Build history of the part. All positions in model axes, mm. Round coordinates to 2 decimals unless told otherwise and drop trailing zeros. Loops run counter-clockwise (first coordinate to the right, second up) from the corner with the lowest first, then second, coordinate; pieces in that order, holes last. Notation, with made-up numbers: (72.5, 63.25) - (80.5, 63.25) arc R14 ccw to (80.5, 82.25) - close; hole circle Ø5 at (-8.5, 4). An arc over 180 degrees is marked (long way). Put each result on its own line as item: value. Start each with the question number.
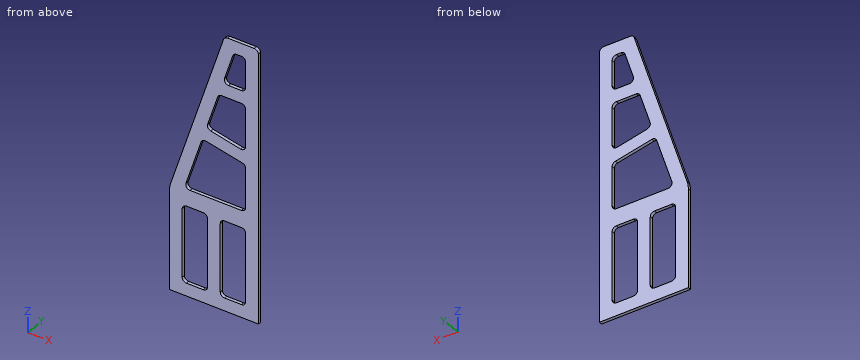
from build123d import *

# Parameters (mm, degrees)
F0_W     = 152.4
F0_H     = 457.2
F1_DEPTH = 19.05
F2_R     = 25.4
F4_R     = 152.4


# Not quite as in the source:
# - two fillets or chamfers of one size are made in one step


with BuildPart() as f1:
    # F0 (on Front) → F1 (new body)
    with BuildSketch(Plane.XZ):
        Polygon((266.7, -812.8), (266.7, 812.8), (63.5, 812.8), (-266.7, -203.2), (-266.7, -812.8), align=None)
        with Locations((-114.3, -508)):
            Rectangle(F0_W, F0_H, mode=Mode.SUBTRACT)
        with Locations((114.3, -508)):
            Rectangle(F0_W, F0_H, mode=Mode.SUBTRACT)
        Polygon((190.5, -177.8), (-178.3216873813, -177.8), (-79.2616873813, 127), (-69.7940460934, 156.1312039627), (190.5, 101.6), align=None, mode=Mode.SUBTRACT)
        Polygon((190.5, 457.2), (190.5, 228.6), (190.5, 177.8), (-46.2416873813, 228.6), (28.0533126187, 457.2), align=None, mode=Mode.SUBTRACT)
        Polygon((118.67604537, 736.6), (190.5, 736.6), (190.5, 533.4), (52.8183126187, 533.4), align=None, mode=Mode.SUBTRACT)
    extrude(amount=F1_DEPTH)

    # F2
    f2_edges = [f1.edges().sort_by_distance(p)[0] for p in [
        (28.053313, -9.525, 457.2),
        (-178.321687, -9.525, -177.8),
        (-190.5, -9.525, -279.4),
        (38.1, -9.525, -279.4),
        (-38.1, -9.525, -279.4),
        (190.5, -9.525, -279.4),
        (190.5, -9.525, 457.2),
        (190.5, -9.525, -177.8),
        (-190.5, -9.525, -736.6),
        (38.1, -9.525, -736.6),
        (-38.1, -9.525, -736.6),
        (190.5, -9.525, -736.6),
        (190.5, -9.525, 533.4),
        (266.7, -9.525, 812.8),
        (52.818313, -9.525, 533.4),
        (190.5, -9.525, 736.6),
        (118.676045, -9.525, 736.6),
        (190.5, -9.525, 177.8),
        (-46.241687, -9.525, 228.6),
        (-69.794046, -9.525, 156.131204),
        (190.5, -9.525, 101.6),
        (63.5, -9.525, 812.8),
    ]]
    fillet(f2_edges, radius=F2_R)

    # F4
    f4_edges = [f1.edges().sort_by_distance(p)[0] for p in [
        (-266.7, -9.525, -203.2),
    ]]
    fillet(f4_edges, radius=F4_R)


solid = f1.part
Item 1: Slice it at A-A (z = -631.5). Give the cut face in (x, y).
Item 2: Slice it at C-C (y = -13). Give the number of separate pieces and of enclosed holes in the cut face, plus the area to 3 significant figures.
Item 3: Slice it at D-D (z = 37.5). Give the cut face in (x, y), plus the area to 3 significant figures.
Item 4: Slice it at B-B (z = 650). Give the cut face in (x, y), plus the area to 3 significant figures.
Item 5: Drop flat-ended pins along their axis: pin 1 Ø9.5 at (y, z) = (-12.5, -84.5) entering from -X; pin 2 Ø8 at (y, z) = (-16.5, 541.5) entering from -X; pin 3 Ø9.5 at (y, z) = (-7.5, 311) entering from -X. Give the stop position or say it passes through.
Item 6: Drill centre lines: probe 1 along X at (y, z) = (-15.5, -486); probe 2 along Z at (x, y) = (150, -13); probe 3 along Z at (x, y) = (157.5, -6.5). Where is each one in solid material? Low to high. Write a range as [from, to].
Computed values:
1. outline: (-266.7, -19.05) - (-190.5, -19.05) - (-190.5, 0) - (-266.7, 0) - close; (-38.1, -19.05) - (38.1, -19.05) - (38.1, 0) - (-38.1, 0) - close; (190.5, -19.05) - (266.7, -19.05) - (266.7, 0) - (190.5, 0) - close
2. separate pieces: 1
2. enclosed holes: 5
2. area: 392,000 mm^2
3. outline: (-188.47, -19.05) - (-108.35, -19.05) - (-108.35, 0) - (-188.47, 0) - close; (190.5, -19.05) - (266.7, -19.05) - (266.7, 0) - (190.5, 0) - close
3. area: 2,980 mm^2
4. outline: (10.59, -19.05) - (90.61, -19.05) - (90.61, 0) - (10.59, 0) - close; (190.5, -19.05) - (266.7, -19.05) - (266.7, 0) - (190.5, 0) - close
4. area: 2,980 mm^2
5. pin 1: stops at x = -229.67
5. pin 2: stops at x = -25.97
5. pin 3: stops at x = -101.13
6. probe 1: x = [-266.7, -190.5], [-38.1, 38.1], [190.5, 266.7]
6. probe 2: z = [-812.8, -736.6], [-279.4, -177.8], [110.08, 186.49], [457.2, 533.4], [736.6, 812.8]
6. probe 3: z = [-812.8, -736.6], [-279.4, -177.8], [108.51, 184.88], [457.2, 533.4], [736.6, 812.8]
